from build123d import *

# Parameters (mm, degrees)
EXTRUDE_1_DEPTH = 10
EXTRUDE_2_DEPTH = 10
EXTRUDE_4_DEPTH = 10
FILLET_1_R      = 7


with BuildPart() as part:
    # 草图2 → 凸台-拉伸1 (new body)
    with BuildSketch(Plane(origin=(0, 0, 0), x_dir=(1, 0, 0), z_dir=(0, 1, 0))):
        Polygon((-20.179491924, 74.951905284), (-5.179491924, 48.97114317), (7.810889132, 56.47114317), (4.060889132, 62.966333699), (20.207259422, 62.966333699), (44.426814855, 48.983166849), (52.5, 35), (45, 35), (45, 20), (75, 20), (75, 35), (67.5, 35), (49.627132403, 65.956714755), (83.660254038, 124.903810568), (66.339745962, 134.903810568), (32.306624327, 75.956714755), (-3.439110868, 75.956714755), (-7.189110868, 82.451905284), align=None)
    extrude(amount=EXTRUDE_1_DEPTH)

    # 草图3 → 凸台-拉伸2 (add)
    with BuildSketch(Plane(origin=(0, 10, 0), x_dir=(1, 0, 0), z_dir=(0, 1, 0))):
        with BuildLine():
            Line((66.339745962, 134.903810568), (59.883306725, 123.720929773))
            ThreePointArc((59.883306725, 123.720929773), (67.5, 116.913429511), (77.2038148, 113.720929773))
            Line((77.2038148, 113.720929773), (83.660254038, 124.903810568))
            Line((83.660254038, 124.903810568), (66.339745962, 134.903810568))
        make_face()
    extrude(amount=EXTRUDE_2_DEPTH)

    # 草图5 → 凸台-拉伸4 (add)
    with BuildSketch(Plane(origin=(0, 10, 0), x_dir=(1, 0, 0), z_dir=(0, 1, 0))):
        Polygon((38.379214965, 52.474750274), (40.879214965, 56.804877293), (28.754859312, 63.804877293), (26.254859312, 59.474750274), align=None)
    extrude(amount=EXTRUDE_4_DEPTH)

    # 圆角1
    fillet_1_edges = [part.edges().sort_by_distance(p)[0] for p in [
        (66.339745962, 10, -134.903810568),
        (83.660254038, 10, -124.903810568),
    ]]
    fillet(fillet_1_edges, radius=FILLET_1_R)


solid = part.part
Design review of the part built by this model. Coordinates are the model's own, in mm. A direction names the side the tool comes from. Coordinates: 2 decimals unless noted, no trailing zeros. Write each loop counter-clockwise with the first axis right and the second up, starting at its lowest first coordinate (ties: lowest second). Pieces come first, ordered by that corner, then holes. Notation, with made-up numbers: (-37, 47) -> (19, 47) arc R9 cw to (19, 64) -> close; hole circle Ø1 at (-7.75, 1.5). An arc over 180 degrees is marked (long way). Write each question's results on one line, items separated by ' | '. Start each with the question number.
(1) Clearance check with flat-ended pins moving along their axes: P1, Ø3, axis at x = 9.5, y = 4, coming from the +Z side; P2, Ø10, axis at y = 11.5, z = -46.5, coming from the -X side; P3, Ø3, axis at y = 3.5, z = -25.5, coming from the -X side. State where each tip first meets the part, or that it passes through.
(2) Take a section at C-C on y = 8. Write out the cut boundary in (x, z), and give its area (3 significant figures).
(3) Take a section at D-D on x = 65.5. Write out the cut boundary in (y, z), and give its area (3 significant figures).
(4) Take a section at A-A on y = 15.5. Write out the cut boundary in (x, z), and give its area (3 significant figures).
(5) For line 1 along Y through (x, z) = (62.5, -116.5); line 2 along Z through (x, y) = (68, 7.5); line 3 along Z through (x, y) = (18, 4), list the stretches that pass through material, from the lowest coordinate up. Write a range as from..to.
(6) Take a section at B-B on x = 51. Write out the cut boundary in (y, z).
(7) Tool access review of faces 1 (the face through (5.962, 4.93, -59.673)), 2 (the face through (45, 5, -28)), 3 (the face through (49, 5, -35)), 4 (the face through (75, 5, -27)): name each direction out of +Z, -Z, +X, -X, +Y, -Y from which nothing blocks a thin tool from reaching the whole face with its end or side.
(8) The part is to be moulded in two halves that separate along X. For faces 5 (the face through (34.902, 14.93, -60.256)), 6 (the face through (48.4, 4.9, -42.1)), 7 (the face through (1.225, 4.93, -52.669)), say which applies: pulls with the +X half, pulls with the -X half, needs draft (parallel to the pull), parting line crosses it, or undercut.
Results found:
1) P1: stops at z = -62.97 | P2: stops at x = -6.51 | P3: stops at x = 45
2) outline: (-20.18, -74.95) -> (-7.19, -82.45) -> (-3.44, -75.96) -> (32.31, -75.96) -> (62.84, -128.84) arc R7 ccw to (72.4, -131.4) -> (77.6, -128.4) arc R7 ccw to (80.16, -118.84) -> (49.63, -65.96) -> (67.5, -35) -> (75, -35) -> (75, -20) -> (45, -20) -> (45, -35) -> (52.5, -35) -> (44.43, -48.98) -> (20.21, -62.97) -> (4.06, -62.97) -> (7.81, -56.47) -> (-5.18, -48.97) -> close | area: 3,330 mm2
3) outline: (0, -131.46) -> (20, -131.46) -> (20, -118.2) -> (10, -118.2) -> (10, -93.45) -> (0, -93.45) -> close; (0, -38.46) -> (10, -38.46) -> (10, -20) -> (0, -20) -> close | area: 697 mm2
4) outline: (26.25, -59.47) -> (28.75, -63.8) -> (40.88, -56.8) -> (38.38, -52.47) -> close; (59.88, -123.72) -> (62.84, -128.84) arc R7 ccw to (72.4, -131.4) -> (77.6, -128.4) arc R7 ccw to (80.16, -118.84) -> (77.2, -113.72) arc R25 ccw to start | area: 335 mm2
5) line 1: y = 0..10 | line 2: z = -132.28..-97.78, -35..-20 | line 3: z = -75.96..-62.97
6) outline: (0, -108.33) -> (10, -108.33) -> (10, -68.33) -> (0, -68.33) -> close; (0, -63.58) -> (10, -63.58) -> (10, -37.6) -> (0, -37.6) -> close; (0, -35) -> (10, -35) -> (10, -20) -> (0, -20) -> close
7) face 1: +Y, -Y | face 2: +Z, -X, +Y, -Y | face 3: -X, +Y, -Y | face 4: +Z, +X, +Y, -Y
8) face 5: pulls with the +X half | face 6: pulls with the -X half | face 7: undercut
